Here's how the part is built. I have some questions about the finished solid (model axes, mm). Face numbers are marked on the shaded views. Round coordinates to 2 decimals unless told otherwise and drop trailing zeros. Put each result on its own line as item: value. Start each with the question number.
1. I need wall thicknesses on probe 1 along X at (y, z) = (8.75, -0.25); probe 2 along X at (y, z) = (17, -1.25); probe 3 along X at (y, z) = (2, -1.25). Which ranges of each line are inside material? Lowest first, please. Write a range as from..to.
2. We'd pull the mould along X, two halves only. Please class the marked faces 1 and 2: +X half, -X half, draft (parallel to the pull), parting line (faces both ways), or undercut.
3. For pin 1 (2.5 mm diameter, centred on x = -1.5, y = 11.5, fed in from +Z); pin 2 (1.5 mm diameter, centred on y = 7, z = -1, fed in from +X); pin 3 (1.5 mm diameter, centred on y = 16.5, z = -6.5, fed in from -X), each with a flat end and sliding along its axis, tell me the tip position at first contact or that it passes through.
```python
from build123d import *

# Parameters (mm, degrees)
SKETCH2_W          = 21.920038039
SKETCH2_H          = 22.914873095
CUT_EXTRUDE1_DEPTH = 9


with BuildPart() as part:
    # Sketch1 → Revolve1 (revolve)
    with BuildSketch(Plane.XY):
        with BuildLine():
            Line((6.5, 0), (9, 0))
            add(Edge.make_bspline(
                [(0, 20.35), (1.675966842, 20.428176516), (5.66035993, 19.372470149), (8.740520085, 10.941984052), (8.794057121, 4.785623995), (9, 0)],
                knots=[0, 0, 0, 0, 0.209086974, 0.440428739, 1, 1, 1, 1], degree=3))
            Line((0, 20.35), (0, 17.85))
            add(Edge.make_bspline(
                [(0, 17.85), (1.248468613, 18.003104069), (3.434295374, 16.83334968), (6.617297319, 10.514055415), (6.220398856, 4.532307189), (6.5, 0)],
                knots=[0, 0, 0, 0, 0.174730572, 0.328981961, 1, 1, 1, 1], degree=3))
        make_face()
    revolve(axis=Axis((0, 24.080193906, 0), (0, -1, 0)))

    # Sketch2 → Cut-Extrude1 (cut)
    with BuildSketch(Plane.XY.offset(9)):
        with Locations((-0.139254467, 10.620448961)):
            Rectangle(SKETCH2_W, SKETCH2_H)
    extrude(amount=-CUT_EXTRUDE1_DEPTH, mode=Mode.SUBTRACT)

    # Loft1: read off the stored shape, not the designer's step
    # Loft1: loft between two sections, ruled curve by curve
    loft1_from = [
        Edge.make_bspline([(0, 1.344428361, -7.62463212), (10.784005956, 1.344428361, -7.62463212), (10.784005956, 18.932107275, -4.523449799), (0, 18.932107275, -4.523449799), (-10.784005956, 18.932107275, -4.523449799), (-10.784005956, 1.344428361, -7.62463212), (0, 1.344428361, -7.62463212)], [0, 0, 0, 0, 0.5, 0.5, 0.5, 1, 1, 1, 1], 3, [1, 0.333333333, 0.333333333, 1, 0.333333333, 0.333333333, 1]),
    ]
    loft1_to = [
        Edge.make_bspline([(0.012725843, 6.000020243, -0.2), (8.012685357, 6.02547193, -0.2), (7.98723367, 14.025431443, -0.2), (-0.012725843, 13.999979757, -0.2), (-8.012685357, 13.97452807, -0.2), (-7.98723367, 5.974568557, -0.2), (0.012725843, 6.000020243, -0.2)], [0, 0, 0, 0, 0.5, 0.5, 0.5, 1, 1, 1, 1], 3, [1, 0.333333333, 0.333333333, 1, 0.333333333, 0.333333333, 1]),
    ]
    loft1 = Solid(Shell([*[Face.make_surface_from_curves(loft1_from[k], loft1_to[k]) for k in range(1)], Face(Wire(loft1_from)), Face(Wire(loft1_to))]))
    add(loft1)


solid = part.part
```
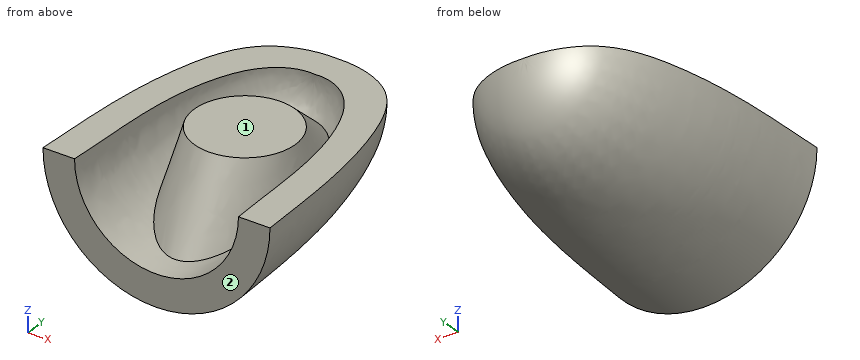
Verdict:
1. probe 1: x = -8.46..-6.03, -3.81..3.81, 6.03..8.46
1. probe 2: x = -6.19..-2.4, 2.4..6.19
1. probe 3: x = -8.83..-6.28, 6.28..8.83
2. face 1: undercut
2. face 2: draft
3. pin 1: stops at z = -0.2
3. pin 2: stops at x = 8.67
3. pin 3: stops at x = -3.34
